Design review of the part built by this model. Coordinates are the model's own, in mm. Face numbers are marked on the shaded views. A direction names the side the tool comes from. Coordinates: 2 decimals unless noted, no trailing zeros. Write each loop counter-clockwise with the first axis right and the second up, starting at its lowest first coordinate (ties: lowest second). Pieces come first, ordered by that corner, then holes.
Q1. Clearance check with flat-ended pins moving along their axes: pin 1 Ø3 at (x, z) = (-7.5, -10) entering from +Y; pin 2 Ø3 at (y, z) = (-4.5, -22.5) entering from -X; pin 3 Ø1 at (y, z) = (-11, -10) entering from -X; pin 4 Ø5.5 at (x, y) = (-10, 0) entering from -Z (1 decimal). State where each tip first meets the part, or that it passes through.
Q2. Add section B-B, the plane x = 0. Give the boundary of the cut face in (y, z), plus the area to 3 significant figures.
Q3. Add section D-D, the plane z = -22.25. Give the boundary of the cut face in (x, y), plus the area to 3 significant figures.
Q4. The part is to be moulded in two halves that separate along X. For the marked faces 3, 4 and 5, say which applies: +X half, -X half, draft (parallel to the pull), parting line (faces both ways), or undercut.
Q5. Machinability: for the marked faces 1 and 2, which of the approach directions +Z, -Z, +X, -X, +Y, -Y give a long, thin tool a straight path to every point of the face, cutting with its end or side? Answer none if there is none.
Q6. Add section C-C, the plane y = 0. Give the boundary of the cut face in (x, z).
Q7. Add section A-A, the plane z = -4.25. Give the boundary of the cut face in (x, y).
Q8. To check wall thickness, follow probe 1 along Y at (x, z) = (0, -4.5); probe 2 along Y at (x, z) = (3.5, -6.25); probe 3 along Z at (x, y) = (-17, -8). State the ranges of each line that lie inside material, in increasing order.
from build123d import *

# Parameters (mm, degrees)
F2_R     = 5
F3_DEPTH = 25.001
F4_R     = 3
F5_DEPTH = 25.001


with BuildPart() as f1:
    # F0 (on Front) → F1 (revolve)
    with BuildSketch(Plane.XZ):
        Polygon((20, 0), (0, 0), (0, -25), (15, -25), (15, -1), (17.1, -1), (17.1, -12), (20, -12), align=None)
    revolve(axis=Axis((0, 0, -20.761178), (0, 0, -1)))

    # F2 (on Top) → F3 (cut, through all)
    with BuildSketch(Plane.XY):
        Circle(F2_R)
    extrude(amount=-F3_DEPTH, mode=Mode.SUBTRACT)

    # F4 (on face) → F5 (cut, through all)
    with BuildSketch(Plane.XY):
        with Locations((-10, 0)):
            Circle(F4_R)
    extrude(amount=-F5_DEPTH, mode=Mode.SUBTRACT)


solid = f1.part
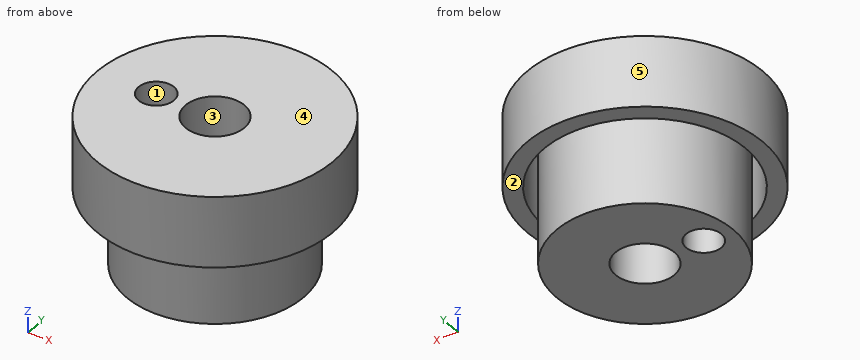
Here are the results:
1. pin 1: stops at y = 19.08
1. pin 2: stops at x = -14.7
1. pin 3: stops at x = -17.02
1. pin 4: passes through
2. outline: (-20, -12) - (-17.1, -12) - (-17.1, -1) - (-15, -1) - (-15, -25) - (-5, -25) - (-5, 0) - (-20, 0) - close; (5, -25) - (15, -25) - (15, -1) - (17.1, -1) - (17.1, -12) - (20, -12) - (20, 0) - (5, 0) - close
2. area: 574 mm2
3. outline: circle Ø30 at (0, 0); hole circle Ø6 at (-10, 0); hole circle Ø10 at (0, 0)
3. area: 600 mm2
4. face 3: undercut
4. face 4: draft
4. face 5: parting line
5. face 1: +Z, -Z
5. face 2: -Z
6. outline: (-20, -12) - (-17.1, -12) - (-17.1, -1) - (-15, -1) - (-15, -25) - (-13, -25) - (-13, 0) - (-20, 0) - close; (-7, -25) - (-5, -25) - (-5, 0) - (-7, 0) - close; (5, -25) - (15, -25) - (15, -1) - (17.1, -1) - (17.1, -12) - (20, -12) - (20, 0) - (5, 0) - close
7. outline: circle Ø40 at (0, 0); circle Ø30 at (0, 0); hole circle Ø34.2 at (0, 0); hole circle Ø6 at (-10, 0); hole circle Ø10 at (0, 0)
8. probe 1: y = -20 to -17.1, -15 to -5, 5 to 15, 17.1 to 20
8. probe 2: y = -19.69 to -16.74, -14.59 to -3.57, 3.57 to 14.59, 16.74 to 19.69
8. probe 3: z = -12 to 0
